Can you work these out from the model? Positions are in its coordinate system, mm. Face numbers are marked on the shaded views. A direction names the side the tool comes from. Coordinates: 2 decimals unless noted, no trailing zeros. Order: outer loops, then holes, each group sorted by start corner. A loop starts at its lowest first (then second) coordinate and runs counter-clockwise, first axis right, second up. Notation, with made-up numbers: (-39, 23) -> (-32, 23) arc R25 ccw to (-32, 43) -> close; hole circle Ø8 at (30, 52.5). An arc over 180 degrees is marked (long way). Answer in a Markdown table with one row per item.
```python
from build123d import *

# Parameters (mm, degrees)
SKETCH1_R           = 40
BOSS_EXTRUDE1_DEPTH = 710
SKETCH2_R           = 60
BOSS_EXTRUDE2_DEPTH = 120
SKETCH3_R           = 60
BOSS_EXTRUDE3_DEPTH = 120
BOSS_EXTRUDE4_DEPTH = 92
BOSS_EXTRUDE5_DEPTH = 92


with BuildPart() as part:
    # Sketch1 → Boss-Extrude1 (new body)
    with BuildSketch(Plane.XY):
        Circle(SKETCH1_R)
    extrude(amount=BOSS_EXTRUDE1_DEPTH)

    # Sketch2 → Boss-Extrude2 (add)
    with BuildSketch(Plane.XY.offset(710)):
        Circle(SKETCH2_R)
    extrude(amount=BOSS_EXTRUDE2_DEPTH)

    # Sketch3 → Boss-Extrude3 (add)
    with BuildSketch(Plane(origin=(0, 0, 0), x_dir=(-1, 0, 0), z_dir=(0, 0, -1))):
        Circle(SKETCH3_R)
    extrude(amount=BOSS_EXTRUDE3_DEPTH)

    # Sketch4 → Boss-Extrude4 (add)
    with BuildSketch(Plane.XY.offset(830)):
        with BuildLine():
            Line((-28.284271247, 10), (-50, 10))
            Line((-50, 10), (-50, -10))
            Line((-50, -10), (-28.284271247, -10))
            ThreePointArc((-28.284271247, -10), (-30, 0), (-28.284271247, 10))
        make_face()
        with BuildLine():
            ThreePointArc((28.284271247, 10), (0, 30), (-28.284271247, 10))
            Line((-28.284271247, 10), (28.284271247, 10))
        make_face()
        with BuildLine():
            Line((28.284271247, 10), (-28.284271247, 10))
            ThreePointArc((-28.284271247, 10), (-30, 0), (-28.284271247, -10))
            Line((-28.284271247, -10), (28.284271247, -10))
            ThreePointArc((28.284271247, -10), (29.56795679, -5.073059362), (30, 0))
            ThreePointArc((30, 0), (29.56795679, 5.073059362), (28.284271247, 10))
        make_face()
        with BuildLine():
            Line((28.284271247, -10), (-28.284271247, -10))
            ThreePointArc((-28.284271247, -10), (0, -30), (28.284271247, -10))
        make_face()
        with BuildLine():
            Line((50, 10), (28.284271247, 10))
            ThreePointArc((28.284271247, 10), (29.56795679, 5.073059362), (30, 0))
            ThreePointArc((30, 0), (29.56795679, -5.073059362), (28.284271247, -10))
            Line((28.284271247, -10), (50, -10))
            Line((50, -10), (50, 10))
        make_face()
    extrude(amount=BOSS_EXTRUDE4_DEPTH)

    # Sketch5 → Boss-Extrude5 (add)
    with BuildSketch(Plane(origin=(0, 0, -120), x_dir=(-1, 0, 0), z_dir=(0, 0, -1))):
        with BuildLine():
            Line((-28.284271247, 10), (28.284271247, 10))
            ThreePointArc((28.284271247, 10), (0, 30), (-28.284271247, 10))
        make_face()
        with BuildLine():
            Line((-50, -10), (-28.284271247, -10))
            ThreePointArc((-28.284271247, -10), (-30, 0), (-28.284271247, 10))
            Line((-28.284271247, 10), (-50, 10))
            Line((-50, 10), (-50, -10))
        make_face()
        with BuildLine():
            Line((-28.284271247, -10), (28.284271247, -10))
            ThreePointArc((28.284271247, -10), (29.56795679, -5.073059362), (30, 0))
            ThreePointArc((30, 0), (29.56795679, 5.073059362), (28.284271247, 10))
            Line((28.284271247, 10), (-28.284271247, 10))
            ThreePointArc((-28.284271247, 10), (-30, 0), (-28.284271247, -10))
        make_face()
        with BuildLine():
            ThreePointArc((-28.284271247, -10), (0, -30), (28.284271247, -10))
            Line((28.284271247, -10), (-28.284271247, -10))
        make_face()
        with BuildLine():
            Line((28.284271247, -10), (50, -10))
            Line((50, -10), (50, 10))
            Line((50, 10), (28.284271247, 10))
            ThreePointArc((28.284271247, 10), (29.56795679, 5.073059362), (30, 0))
            ThreePointArc((30, 0), (29.56795679, -5.073059362), (28.284271247, -10))
        make_face()
    extrude(amount=BOSS_EXTRUDE5_DEPTH)


solid = part.part
```
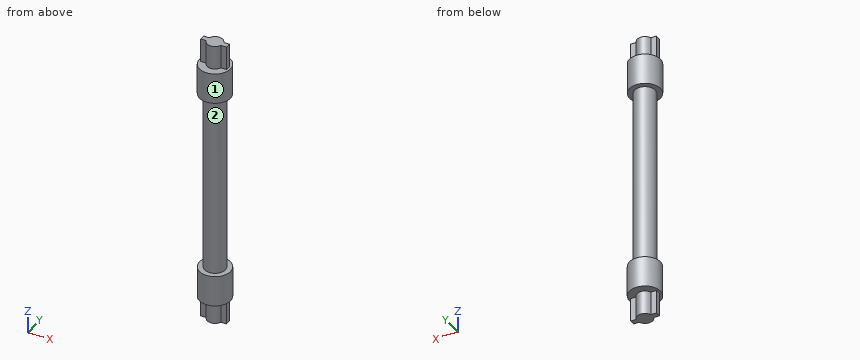
(1) Suppose I cut it at A-A (y = 0). Please give me the cut outline in (x, z), and give its area (3 significant figures).
Response values:
| item | result |
|---|---|
| outline | (-60, -120) -> (-50, -120) -> (-50, -212) -> (50, -212) -> (50, -120) -> (60, -120) -> (60, 0) -> (40, 0) -> (40, 710) -> (60, 710) -> (60, 830) -> (50, 830) -> (50, 922) -> (-50, 922) -> (-50, 830) -> (-60, 830) -> (-60, 710) -> (-40, 710) -> (-40, 0) -> (-60, 0) -> close |
| area | 104,000 mm2 |
(2) Suppose I cut it at B-B (x = -15). Please give me the cut outline in (y, z), and give its area (3 significant figures).
Response values:
| item | result |
|---|---|
| outline | (-58.09, -120) -> (-25.98, -120) -> (-25.98, -212) -> (25.98, -212) -> (25.98, -120) -> (58.09, -120) -> (58.09, 0) -> (37.08, 0) -> (37.08, 710) -> (58.09, 710) -> (58.09, 830) -> (25.98, 830) -> (25.98, 922) -> (-25.98, 922) -> (-25.98, 830) -> (-58.09, 830) -> (-58.09, 710) -> (-37.08, 710) -> (-37.08, 0) -> (-58.09, 0) -> close |
| area | 90,100 mm2 |
(3) Suppose I cut it at C-C (z = 696). Please give me the cut outline in (x, y), and give its area (3 significant figures).
Response values:
| item | result |
|---|---|
| outline | circle Ø80 at (0, 0) |
| area | 5,030 mm2 |
(4) I need wall thicknesses on line 1 (Z direction, x = 49.5, y = 9); line 2 (Z direction, x = 46, y = 30); line 3 (Y direction, x = -0.5, z = 156.5). Which ranges of each line are inside material? Lowest first, please. Write a range as [from, to].
Response values:
| item | result |
|---|---|
| line 1 | [-212, 0], [710, 922] |
| line 2 | [-120, 0], [710, 830] |
| line 3 | [-40, 40] |
(5) On a 3-axis mill with a long thin cutter (end or side, diameter ignored), from which of +Z, -Z, +X, -X, +Y, -Y can I reach the whole of each face in a straight line? I mean the marked faces 1 and 2. Say none if no direction works.
Response values:
| item | result |
|---|---|
| face 1 | +Z, -Z |
| face 2 | none |
(6) Suppose I cut it at D-D (z = -89). Please give me the cut outline in (x, y).
Response values:
| item | result |
|---|---|
| outline | circle Ø120 at (0, 0) |
(7) Will these pins go through, and if not, where does the flat tip stop? pin 1 Ø17.5 at (x, z) = (42.5, -169.5) entering from -Y; pin 2 Ø10 at (y, z) = (-4, -180) entering from -X; pin 3 Ø11 at (x, z) = (38.5, -149) entering from +Y.
Response values:
| item | result |
|---|---|
| pin 1 | y = -10 |
| pin 2 | x = -50 |
| pin 3 | y = 10 |
